Design review of the part shown in the three views and the two pictorial views. Dimensions are in mm from the part's minimum x, y and z. Give positions to 0.01 mm unless a question says otherwise; leave off trailing zeros. Loops run counter-clockwise (first coordinate to the right, second up) from the corner with the lowest first, then second, coordinate; pieces in that order, holes last.
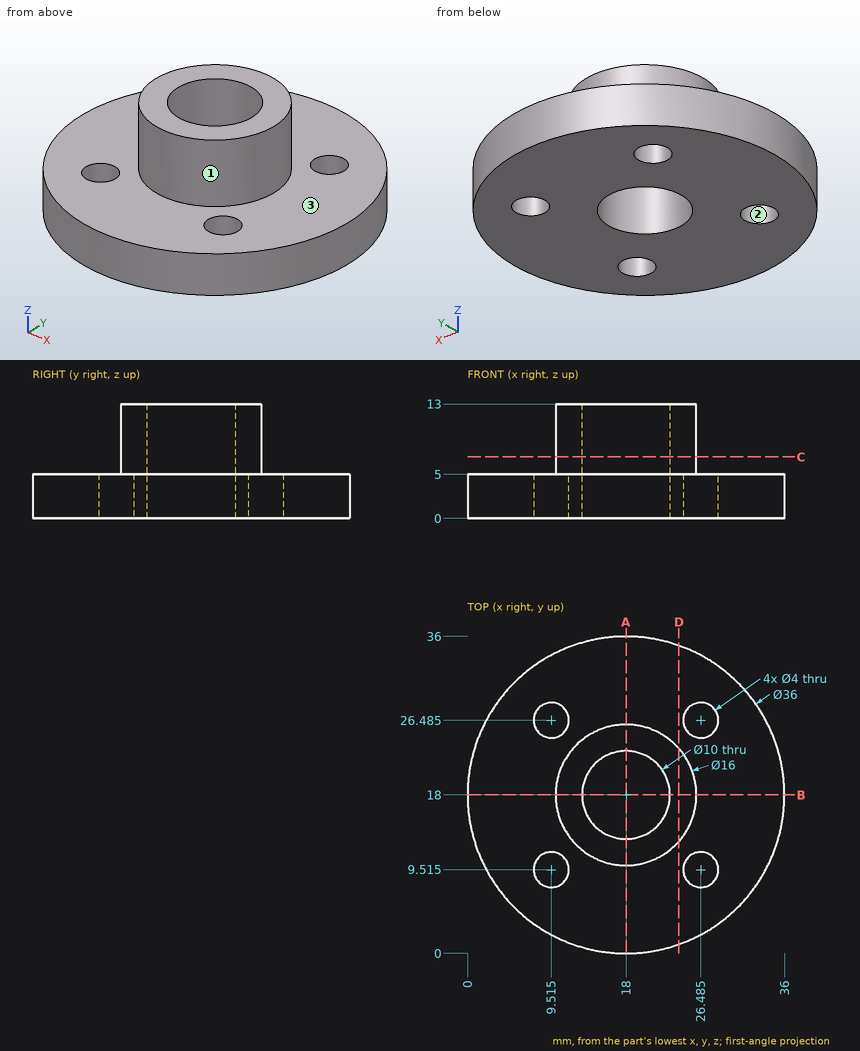
Q1. Take a section at A-A (x = 18). Give the boundary of the cut face in (y, z), plus the area to 3 significant figures.
Results:
outline: (0, 0) - (13, 0) - (13, 13) - (10, 13) - (10, 5) - (0, 5) - close; (23, 0) - (36, 0) - (36, 5) - (26, 5) - (26, 13) - (23, 13) - close
area: 178 mm2
Q2. Draft analysis for pull direction X (two halves, no side actions). For the marked faces 1, 2 and 3, state which applies: pulls with the +X half, pulls with the -X half, needs draft (parallel to the pull), parting line crosses it, or undercut.
Results:
face 1: parting line crosses it
face 2: undercut
face 3: needs draft
Q3. Take a section at C-C (z = 7). Give the boundary of the cut face in (x, y).
Results:
outline: circle Ø16 at (18, 18); hole circle Ø10 at (18, 18)
Q4. Take a section at D-D (x = 24). Give the boundary of the cut face in (y, z), plus the area to 3 significant figures.
Results:
outline: (1.03, 0) - (34.97, 0) - (34.97, 5) - (23.29, 5) - (23.29, 13) - (12.71, 13) - (12.71, 5) - (1.03, 5) - close
area: 254 mm2
Q5. Insertion check: pin 1 (4.5 mm diameter, centred on x = 9.51, y = 26.49, fed in from +Z); pin 2 (3 mm diameter, centred on y = 9.5, z = 8, fed in from +X); pin 3 (1 mm diameter, centred on x = 24.5, z = 1.5, fed in from +Y). Each pin has a flat end and moves straight along its axis. Give the tip position at first contact, or say it passes through.
Results:
pin 1: stops at z = 5
pin 2: stops at x = 21.87
pin 3: stops at y = 34.97
Q6. Wall thickness on line 1 (X direction, y = 26.5, z = 1.75) (1 decimal); line 2 (X direction, y = 26, z = 2.25) (1 decimal); line 3 (Z direction, x = 17.5, y = 6.5): over which ranges is each line inside the solid? List them lowest first.
Results:
line 1: x = 2.1 to 7.5, 11.5 to 24.5, 28.5 to 33.9
line 2: x = 1.9 to 7.6, 11.5 to 24.5, 28.4 to 34.1
line 3: z = 0 to 5
